For this review, take the finished solid that the model builds, in its own axes (mm). Face numbers are marked on the shaded views. Coordinates: 2 decimals unless noted, no trailing zeros. Write each loop counter-clockwise with the first axis right and the second up, starting at its lowest first coordinate (ties: lowest second). Pieces come first, ordered by that corner, then holes.
```python
from build123d import *

# Parameters (mm, degrees)
SKETCH1_R           = 16.4
SKETCH1_R_2         = 2.15
BOSS_EXTRUDE1_DEPTH = 43.15
SKETCH6_R           = 1
CUT_EXTRUDE1_DEPTH  = 5


with BuildPart() as part:
    # Sketch1 → Boss-Extrude1 (new body)
    with BuildSketch(Plane.XY):
        with BuildLine():
            Line((-15.5, -20), (15.5, -20))
            ThreePointArc((15.5, -20), (18.681980515, -18.681980515), (20, -15.5))
            Line((20, -15.5), (20, 15.5))
            ThreePointArc((20, 15.5), (18.681980515, 18.681980515), (15.5, 20))
            Line((15.5, 20), (-15.5, 20))
            ThreePointArc((-15.5, 20), (-18.681980515, 18.681980515), (-20, 15.5))
            Line((-20, 15.5), (-20, -15.5))
            ThreePointArc((-20, -15.5), (-18.681980515, -18.681980515), (-15.5, -20))
        make_face()
        Circle(SKETCH1_R, mode=Mode.SUBTRACT)
        with Locations((-15.5, 15.5)):
            Circle(SKETCH1_R_2, mode=Mode.SUBTRACT)
        with Locations((15.5, 15.5)):
            Circle(SKETCH1_R_2, mode=Mode.SUBTRACT)
        with Locations((15.5, -15.5)):
            Circle(SKETCH1_R_2, mode=Mode.SUBTRACT)
        with Locations((-15.5, -15.5)):
            Circle(SKETCH1_R_2, mode=Mode.SUBTRACT)
    extrude(amount=BOSS_EXTRUDE1_DEPTH)

    # Sketch5 → Cut-Revolve1 (revolve, cut)
    with BuildSketch(Plane(origin=(0, 0, 0), x_dir=(1, 0, 0), z_dir=(0, 1, 0)), mode=Mode.PRIVATE) as cut_revolve1_sk:
        Polygon((16.4, -3.1), (17, -2.5), (17.75, 0), (16.4, 0), align=None)
    cut_revolve1 = revolve(cut_revolve1_sk.sketch.rotate(Axis((0, 0, -2.15), (0, 0, 1)), 180), axis=Axis((0, 0, -2.15), (0, 0, 1)), mode=Mode.SUBTRACT)

    # Mirror1: Cut-Revolve1 across plane
    add(cut_revolve1.mirror(Plane(origin=(0, 0, 21.575), x_dir=(1, 0, 0), z_dir=(0, 0, -1))), mode=Mode.SUBTRACT)

    # Sketch6 → Cut-Extrude1 (cut)
    with BuildSketch(Plane.XY.offset(43.15)):
        with Locations((-11, 17)):
            Circle(SKETCH6_R)
        with Locations(Location((17, -11, 0), (0, 0, 180))):
            Circle(SKETCH6_R)
    extrude(amount=-CUT_EXTRUDE1_DEPTH, mode=Mode.SUBTRACT)


solid = part.part
```
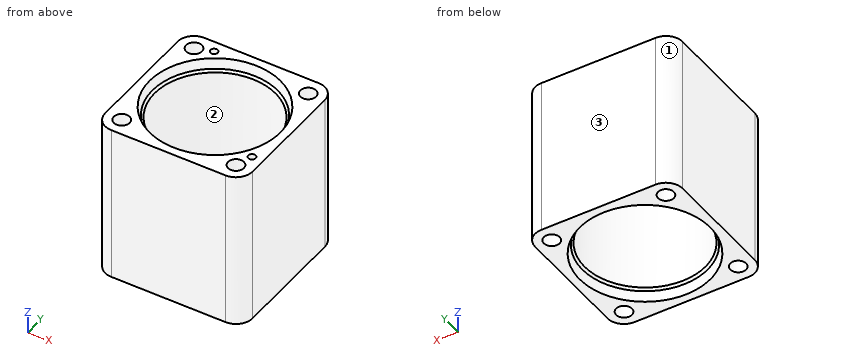
Q1. Add section A-A (x = 0). State the section outline as (y, z) points, then the cut area to 3 significant figures.
Ans:
outline: (-20, 0) - (-17.75, 0) - (-17, 2.5) - (-16.4, 3.1) - (-16.4, 40.05) - (-17, 40.65) - (-17.75, 43.15) - (-20, 43.15) - close; (16.4, 3.1) - (17, 2.5) - (17.75, 0) - (20, 0) - (20, 43.15) - (17.75, 43.15) - (17, 40.65) - (16.4, 40.05) - close
area: 300 mm2
Q2. Clearance check with flat-ended pins moving along their axes: pin 1 Ø2 at (x, y) = (16.5, -11) entering from +Z; pin 2 Ø3.5 at (x, y) = (15.5, 15.5) entering from -Z; pin 3 Ø1.2 at (x, y) = (-11, 17) entering from +Z. State where each tip first meets the part, or that it passes through.
Ans:
pin 1: stops at z = 43.15
pin 2: passes through
pin 3: stops at z = 38.15
Q3. Draft analysis for pull direction X (two halves, no side actions). For the marked faces 1, 2 and 3, state which applies: +X half, -X half, draft (parallel to the pull), parting line (faces both ways), or undercut.
Ans:
face 1: -X half
face 2: undercut
face 3: draft
Q4. Add section B-B (z = 34.5). State the section outline as (x, y) points.
Ans:
outline: (-20, -15.5) arc R4.5 ccw to (-15.5, -20) - (15.5, -20) arc R4.5 ccw to (20, -15.5) - (20, 15.5) arc R4.5 ccw to (15.5, 20) - (-15.5, 20) arc R4.5 ccw to (-20, 15.5) - close; hole circle Ø4.3 at (-15.5, -15.5); hole circle Ø4.3 at (-15.5, 15.5); hole circle Ø32.8 at (0, 0); hole circle Ø4.3 at (15.5, -15.5); hole circle Ø4.3 at (15.5, 15.5)
Q5. Add section C-C (y = 14.5). Give the number of separate pieces and of enclosed holes in the cut face, then the cut area to 3 significant figures.
Ans:
separate pieces: 4
enclosed holes: 0
area: 716 mm2
Q6. For probe 1 along X at (y, z) = (-15, 33); probe 2 along X at (y, z) = (-11, 40.4); probe 3 along X at (y, z) = (-11, 41), list the stretches that pass through material, from the lowest coordinate up.
Ans:
probe 1: x = -20 to -17.59, -13.41 to -6.63, 6.63 to 13.41, 17.59 to 20
probe 2: x = -20 to -12.63, 12.63 to 16, 18 to 20
probe 3: x = -20 to -13.1, 13.1 to 16, 18 to 20
